The model under review builds one solid part; all positions refer to its coordinate system, in mm. A direction names the side the tool comes from. Round coordinates to 2 decimals unless told otherwise and drop trailing zeros. Order: outer loops, then holes, each group sorted by start corner. A loop starts at its lowest first (then second) coordinate and runs counter-clockwise, first axis right, second up.
1) To check wall thickness, follow L1, parallel to X at y = 1.5, z = -13; L2, parallel to X at y = 2, z = 18.5; L3, parallel to X at y = 3.3, z = 10. State the ranges of each line that lie inside material, in increasing order.
2) Mouldability with a two-part tool opening along Z and no side actions: class faces 6 (the face through (75, 2, -44)), 7 (the face through (10.14, 2.465, 27.854)), 8 (the face through (64, 2, 14)), 9 (the face through (5, 2, -12)) as pulls with the +Z half, pulls with the -Z half, needs draft (parallel to the pull), parting line crosses it, or undercut.
3) Consider section C-C (z = -2). Give the boundary of the cut face in (x, y), then the cut area to 3 significant figures.
4) Machinability: for faces 1 (the face through (20, 2, 40)), 2 (the face through (60, 2, -39)), 3 (the face through (27, 2, 0)), 4 (the face through (67, 2, 39)), 5 (the face through (20, 2, -39)), which of the approach directions +Z, -Z, +X, -X, +Y, -Y give a long, thin tool a straight path to every point of the face, cutting with its end or side? Answer none if there is none.
5) Clearance check with flat-ended pins moving along their axes: P1, Ø5, axis at x = 5, z = -10, coming from the +Y side; P2, Ø5, axis at x = 50, z = 12, coming from the -Y side; P3, Ø4, axis at x = 72.5, y = 2, coming from the -Z side; P4, Ø2.5, axis at x = 62.5, y = 3, coming from the -Z side. State where each tip first meets the part, or that it passes through.
6) Consider section D-D (z = -40). Give the boundary of the cut face in (x, y).
7) Consider section A-A (z = 10). Give the boundary of the cut face in (x, y), then the cut area to 3 significant figures.
8) Consider section B-B (x = 64). Give the boundary of the cut face in (y, z), then the cut area to 3 significant figures.
from build123d import *

# Parameters (mm, degrees)
SKETCH3_R           = 2
SKETCH3_R_2         = 3.5
SKETCH3_W           = 12
SKETCH3_H           = 48
SKETCH3_W_2         = 10
SKETCH3_H_2         = 28
BOSS_EXTRUDE1_DEPTH = 5
SKETCH3_2_R         = 3.5
BOSS_EXTRUDE2_DEPTH = 8


with BuildPart() as part:
    # Sketch3 → Boss-Extrude1 (new body)
    with BuildSketch(Plane(origin=(0, 0, 0), x_dir=(1, 0, 0), z_dir=(0, 1, 0))):
        Polygon((0, -22), (0, 22), (20, 33.547005384), (20, 45.547005384), (40, 45.547005384), (40, 34), (55, 34), (65, 44), (85, 44), (85, 41), (67, 41), (67, 37), (73, 37), (73, 25), (85, 25), (85, 14), (80, 14), (80, -14), (85, -14), (85, -25), (73, -25), (73, -37), (67, -37), (67, -41), (85, -41), (85, -44), (65, -44), (55, -34), (40, -34), (40, -45.547005384), (20, -45.547005384), (20, -33.547005384), align=None)
        with Locations(Location((55, 27, 0), (0, 0, 270))):
            Circle(SKETCH3_R, mode=Mode.SUBTRACT)
        with Locations(Location((30, 40, 0), (0, 0, 270))):
            Circle(SKETCH3_R_2, mode=Mode.SUBTRACT)
        with Locations(Location((5, 10, 0), (0, 0, 270))):
            Circle(SKETCH3_R, mode=Mode.SUBTRACT)
        with Locations(Location((5, -10, 0), (0, 0, 90))):
            Circle(SKETCH3_R, mode=Mode.SUBTRACT)
        with Locations(Location((30, -40, 0), (0, 0, 90))):
            Circle(SKETCH3_R_2, mode=Mode.SUBTRACT)
        with Locations(Location((55, -27, 0), (0, 0, 90))):
            Circle(SKETCH3_R, mode=Mode.SUBTRACT)
        with Locations((33, 0)):
            Rectangle(SKETCH3_W, SKETCH3_H, mode=Mode.SUBTRACT)
        with Locations((64, 0)):
            Rectangle(SKETCH3_W_2, SKETCH3_H_2, mode=Mode.SUBTRACT)
        Polygon((12, 19), (12, -19), (21, -24), (21, 24), align=None, mode=Mode.SUBTRACT)
    extrude(amount=BOSS_EXTRUDE1_DEPTH)

    # Sketch3_2 → Boss-Extrude2 (add)
    with BuildSketch(Plane(origin=(0, 0, 0), x_dir=(1, 0, 0), z_dir=(0, 1, 0))):
        with Locations(Location((30, 40, 0), (0, 0, 270))):
            Circle(SKETCH3_2_R)
        with Locations(Location((30, -40, 0), (0, 0, 90))):
            Circle(SKETCH3_2_R)
    extrude(amount=BOSS_EXTRUDE2_DEPTH)


solid = part.part
Answer below:
1. L1: x = 0 to 12, 21 to 27, 39 to 59, 69 to 80
1. L2: x = 0 to 12, 21 to 27, 39 to 85
1. L3: x = 0 to 3, 7 to 12, 21 to 27, 39 to 59, 69 to 80
2. face 6: pulls with the -Z half
2. face 7: pulls with the +Z half
2. face 8: undercut
2. face 9: undercut
3. outline: (0, 0) - (12, 0) - (12, 5) - (0, 5) - close; (21, 0) - (27, 0) - (27, 5) - (21, 5) - close; (39, 0) - (59, 0) - (59, 5) - (39, 5) - close; (69, 0) - (80, 0) - (80, 5) - (69, 5) - close
3. area: 245 mm2
4. face 1: +Z, -X, +Y, -Y
4. face 2: -Z, +Y, -Y
4. face 3: +Y, -Y
4. face 4: +X, +Y, -Y
4. face 5: -Z, -X, +Y, -Y
5. P1: stops at y = 5
5. P2: stops at y = 0
5. P3: stops at z = -44
5. P4: stops at z = -42.75
6. outline: (20, 0) - (40, 0) - (40, 5) - (33.5, 5) - (33.5, 8) - (26.5, 8) - (26.5, 5) - (20, 5) - close; (61, 0) - (67, 0) - (67, 5) - (61, 5) - close
7. outline: (0, 0) - (3, 0) - (3, 5) - (0, 5) - close; (7, 0) - (12, 0) - (12, 5) - (7, 5) - close; (21, 0) - (27, 0) - (27, 5) - (21, 5) - close; (39, 0) - (59, 0) - (59, 5) - (39, 5) - close; (69, 0) - (80, 0) - (80, 5) - (69, 5) - close
7. area: 225 mm2
8. outline: (0, -43) - (5, -43) - (5, -14) - (0, -14) - close; (0, 14) - (5, 14) - (5, 43) - (0, 43) - close
8. area: 290 mm2
